For this review, take the finished solid that the model builds, in its own axes (mm). Round coordinates to 2 decimals unless told otherwise and drop trailing zeros. Order: outer loops, then holes, each group sorted by start corner. A loop starts at its lowest first (then second) coordinate and runs counter-clockwise, first axis right, second up. Notation, with made-up numbers: M -29.75,-1 L -0.75,-1 A13 cw -0.75,11 Z; hole C 56.25,50 d5. An arc over 180 degrees is marked long. Write item = value, one per line. Start each with the question number.
Autodesk Inventor part; units mm, degrees
ref_plane "Work Plane1" through (4, 0, 0) normal (1, 0, 0) x (0, 1, 0)
ref_plane "XZ Plane" through (0, 0, 0) normal (0, 1, 0) x (-1, 0, 0)
ref_plane "XY Plane" through (0, 0, 0) normal (0, 0, 1) x (1, 0, 0)
sketch "Sketch2" plane through (0, 0, 0) normal (0, 1, 0) x (-1, 0, 0)
  circle A0 centre (0, 0) radius 4
  dimension "d6" = 8
extrude "Extrusion1" add sketch "Sketch2" along normal blind 25
chamfer "Chamfer1" distance 0.5 angle 45 1 edges at (4, 25, 0)
chamfer "Chamfer2" distance 0.5 angle 45 1 edges at (4, 0, 0)
ref_plane "Work Plane1" through (4, 0, 0) normal (1, 0, 0) x (0, 1, 0)
sketch "Sketch3" plane through (4, 0, 0) normal (1, 0, 0) x (0, 1, 0)
  circle A0 centre (3.5, 0) radius 1.25
  circle A1 centre (21.5, 0) radius 1.25
  line L0 (0, -3.5) -> (0, 3.5) construction
  line L1 (2.25, 0) -> (1.3552, 0) construction
  line L2 (22.75, 0) -> (24.5, 0) construction
  line L3 (24.5, -4) -> (24.5, 4) construction
  point P0 (0, 0)
  dimension "d15" = 2.5
  dimension "d16" = 2.5
  dimension "d17" = 18
  dimension "d19" = 3.5
extrude "Extrusion2" cut sketch "Sketch3" against normal blind 25
properties part number "reverse gear crankshaft center rod"
(1) Insertion check: pin 1 (2 mm diameter, centred on y = 3.5, z = 0, fed in from -X); pin 2 (3 mm diameter, centred on y = 21.5, z = 1.5, fed in from +X). Each pin has a flat end and moves straight along its axis. Give the tip position at first contact, or say it passes through.
(2) We need section B-B, the plane x = 0. Write out the cut boundary in (y, z), then the cut area to 3 significant figures.
(3) We need section A-A, the plane z = 0. Write out the cut boundary in (x, y).
(4) For line 1 along Y through (x, z) = (0, 0); line 2 along Z through (x, y) = (0, 3.5); line 3 along Z through (x, y) = (1.5, 3.5), list the stretches that pass through material, from the lowest coordinate up.
(5) Draft analysis for pull direction Z (two halves, no side actions). For faces 1 (the flat face through (0, 0, 0)), 2 (the cylindrical face through (-3.695, 12.332, 1.532)), 3 (the cylindrical face through (0.056, 22.655, -0.479)), state which applies: released by +Z, released by -Z, zero draft, split by the parting line, or undercut.
(6) We need section D-D, the plane y = 3.5. Write out the cut boundary in (x, z).
(7) We need section C-C, the plane y = 16.75. Write out the cut boundary in (x, z), then the cut area to 3 significant figures.
Values:
q1.pin_1 = through
q1.pin_2 = 3.97
q2.outline = M 0,-3.5 L 0.5,-4 L 24.5,-4 L 25,-3.5 L 25,3.5 L 24.5,4 L 0.5,4 L 0,3.5 Z; hole C 3.5,0 d2.5; hole C 21.5,0 d2.5
q2.area = 190 mm²
q3.outline = M -4,0.5 L -3.5,0 L 3.5,0 L 4,0.5 L 4,2.25 L -4,2.25 Z; M -4,4.75 L 4,4.75 L 4,20.25 L -4,20.25 Z; M -4,22.75 L 4,22.75 L 4,24.5 L 3.5,25 L -3.5,25 L -4,24.5 Z
q4.line_1 = 0 to 2.25, 4.75 to 20.25, 22.75 to 25
q4.line_2 = -4 to -1.25, 1.25 to 4
q4.line_3 = -3.71 to -1.25, 1.25 to 3.71
q5.face_1 = zero draft
q5.face_2 = split by the parting line
q5.face_3 = undercut
q6.outline = M -3.8,-1.25 A4 ccw 3.8,-1.25 Z; M -3.8,1.25 L 3.8,1.25 A4 ccw Z
q7.outline = C 0,0 d8
q7.area = 50.3 mm²
